Design review of the part built by this model. Coordinates are the model's own, in mm. Face numbers are marked on the shaded views. A direction names the side the tool comes from. Coordinates: 2 decimals unless noted, no trailing zeros. Write each loop counter-clockwise with the first axis right and the second up, starting at its lowest first coordinate (ties: lowest second). Pieces come first, ordered by that corner, then holes.
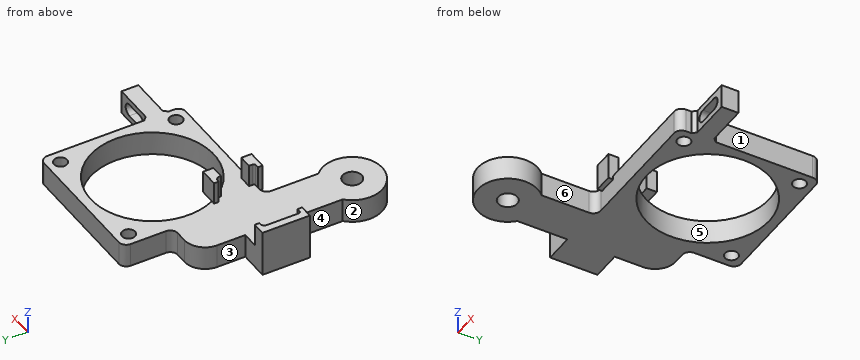
```python
from build123d import *
from OCP.BRepFilletAPI import BRepFilletAPI_MakeFillet

# Parameters (mm, degrees)
SKETCH1_R                 = 2.55
SKETCH1_R_2               = 1.75
SKETCH1_R_3               = 12.5
BOSS_EXTRUDE3_DEPTH       = 6.4
SKETCH1_5_R               = 2.55
BOSS_EXTRUDE2_DEPTH       = 1
CUT_EXTRUDE1_DEPTH        = 10
FILLET2_R                 = 2
CHAMFER2_SIZE             = 1
FILLET1_R                 = 2
SKETCH5_R                 = 16.5
CUT_EXTRUDE2_DEPTH        = 10
SKETCH6_W                 = 4.33
SKETCH6_H                 = 1.25
BOSS_EXTRUDE5_DEPTH       = 6.4
BOSS_EXTRUDE8_DEPTH       = 6
BOSS_EXTRUDE13_DEPTH      = 6
BOSS_EXTRUDE13_DEPTH_BACK = 1
FILLET3_R1                = 1
FILLET3_R2                = 0.5


with BuildPart() as part:
    # Sketch1 → Boss-Extrude3 (new body)
    with BuildSketch(Plane.XY):
        with BuildLine():
            ThreePointArc((-5.55, 5.830951895), (0, -8.05), (5.55, 5.830951895))
            Line((5.55, 5.830951895), (5.55, 20.5))
            Line((5.55, 20.5), (43, 20.5))
            Line((43, 20.5), (43, 25))
            Line((43, 25), (55, 25))
            Line((55, 25), (55, 29.5))
            Line((55, 29.5), (43, 29.5))
            Line((43, 29.5), (43, 58.5))
            Line((43, 58.5), (5, 58.5))
            Line((5, 58.5), (5, 45.05))
            Line((5, 45.05), (0, 45.05))
            ThreePointArc((0, 45.05), (-3.924442636, 43.424442636), (-5.55, 39.5))
            Line((-5.55, 39.5), (-5.55, 5.830951895))
        make_face()
        Circle(SKETCH1_R, mode=Mode.SUBTRACT)
        with Locations((39.5, 24)):
            Circle(SKETCH1_R_2, mode=Mode.SUBTRACT)
        with Locations((8.5, 55)):
            Circle(SKETCH1_R_2, mode=Mode.SUBTRACT)
        with Locations((24, 39.5)):
            Circle(SKETCH1_R_3, mode=Mode.SUBTRACT)
        with Locations((39.5, 55)):
            Circle(SKETCH1_R_2, mode=Mode.SUBTRACT)
    extrude(amount=BOSS_EXTRUDE3_DEPTH)

    # Sketch1<5> → Boss-Extrude2 (add)
    # profile 1 of 2: a face of its own
    with BuildSketch(Plane.XY):
        with BuildLine():
            Line((-5.55, 5.830951895), (-5.55, 0))
            ThreePointArc((-5.55, 0), (0, -5.55), (5.55, 0))
            Line((5.55, 0), (5.55, 5.830951895))
            ThreePointArc((5.55, 5.830951895), (0, 8.05), (-5.55, 5.830951895))
        make_face()
        Circle(SKETCH1_5_R, mode=Mode.SUBTRACT)
    # profile 2 of 2: a face of its own
    with BuildSketch(Plane.XY):
        with BuildLine():
            ThreePointArc((5.55, 0), (0, -5.55), (-5.55, 0))
            Line((-5.55, 0), (-5.55, 5.830951895))
            ThreePointArc((-5.55, 5.830951895), (-3.172144385, -7.398648525), (8.05, 0))
            ThreePointArc((8.05, 0), (7.398648525, 3.172144385), (5.55, 5.830951895))
            Line((5.55, 5.830951895), (5.55, 0))
        make_face()
    extrude(amount=BOSS_EXTRUDE2_DEPTH)

    # Sketch3 → Cut-Extrude1 (cut)
    with BuildSketch(Plane(origin=(0, 29.5, 0), x_dir=(1, 0, 0), z_dir=(0, 1, 0))):
        with BuildLine():
            Line((46.5, -1.55), (51.5, -1.55))
            ThreePointArc((51.5, -1.55), (53.15, -3.2), (51.5, -4.85))
            Line((51.5, -4.85), (46.5, -4.85))
            ThreePointArc((46.5, -4.85), (44.85, -3.2), (46.5, -1.55))
        make_face()
    extrude(amount=-CUT_EXTRUDE1_DEPTH, mode=Mode.SUBTRACT)

    # Fillet2
    fillet2_edges = [part.edges().sort_by_distance(p)[0] for p in [
        (5.55, 20.5, 3.2),
        (5, 45.05, 3.2),
    ]]
    fillet(fillet2_edges, radius=FILLET2_R)

    # Chamfer2
    chamfer2_edges = [part.edges().sort_by_distance(p)[0] for p in [
        (43, 29.5, 3.2),
        (43, 25, 3.2),
    ]]
    chamfer(chamfer2_edges, length=CHAMFER2_SIZE)

    # Fillet1
    fillet1_edges = [part.edges().sort_by_distance(p)[0] for p in [
        (43, 20.5, 3.2),
        (5, 58.5, 3.2),
        (43, 58.5, 3.2),
    ]]
    fillet(fillet1_edges, radius=FILLET1_R)

    # Sketch5 → Cut-Extrude2 (cut)
    with BuildSketch(Plane.XY.offset(6.4)):
        with Locations((24, 39.5)):
            Circle(SKETCH5_R)
    extrude(amount=-CUT_EXTRUDE2_DEPTH, mode=Mode.SUBTRACT)

    # Sketch6 → Boss-Extrude5 (add)
    with BuildSketch(Plane.XY.offset(6.4)):
        with Locations((-7.715, 31.325)):
            Rectangle(SKETCH6_W, SKETCH6_H)
        with BuildLine():
            Line((-5.55, 24.637668909), (-5.55, 30.45))
            Line((-5.55, 30.45), (-10.13, 30.45))
            ThreePointArc((-10.13, 30.45), (-10.837106781, 30.157106781), (-11.13, 29.45))
            Line((-11.13, 29.45), (-11.13, 21.25))
            ThreePointArc((-11.13, 21.25), (-10.983553391, 20.896446609), (-10.63, 20.75))
            Line((-10.63, 20.75), (-5.55, 20.75))
            Line((-5.55, 20.75), (-5.55, 21.862331091))
            ThreePointArc((-5.55, 21.862331091), (-7.525, 23.25), (-5.55, 24.637668909))
        make_face()
        with BuildLine():
            Line((-10.13, 30.45), (-5.55, 30.45))
            Line((-5.55, 30.45), (-5.55, 30.7))
            Line((-5.55, 30.7), (-9.88, 30.7))
            Line((-9.88, 30.7), (-11.38, 30.7))
            Line((-11.38, 30.7), (-11.38, 20.5))
            Line((-11.38, 20.5), (-9.88, 20.5))
            Line((-9.88, 20.5), (-5.55, 20.5))
            Line((-5.55, 20.5), (-5.55, 20.75))
            Line((-5.55, 20.75), (-10.63, 20.75))
            ThreePointArc((-10.63, 20.75), (-10.983553391, 20.896446609), (-11.13, 21.25))
            Line((-11.13, 21.25), (-11.13, 29.45))
            ThreePointArc((-11.13, 29.45), (-10.837106781, 30.157106781), (-10.13, 30.45))
        make_face()
        Polygon((-11.38, 30.7), (-9.88, 30.7), (-9.88, 31.95), (-13.38, 31.95), (-13.38, 19.25), (-9.88, 19.25), (-9.88, 20.5), (-11.38, 20.5), align=None)
        with Locations((-7.715, 19.875)):
            Rectangle(SKETCH6_W, SKETCH6_H)
        with BuildLine():
            Line((-5.55, 21.862331091), (-5.55, 24.637668909))
            ThreePointArc((-5.55, 24.637668909), (-7.525, 23.25), (-5.55, 21.862331091))
        make_face()
        with BuildLine():
            ThreePointArc((-4.575, 23.25), (-4.843118689, 24.09797553), (-5.55, 24.637668909))
            Line((-5.55, 24.637668909), (-5.55, 21.862331091))
            ThreePointArc((-5.55, 21.862331091), (-4.843118689, 22.40202447), (-4.575, 23.25))
        make_face()
    extrude(amount=-BOSS_EXTRUDE5_DEPTH)

    # Sketch6<4> → Boss-Extrude8 (add)
    with BuildSketch(Plane.XY.offset(6.4)):
        Polygon((-9.88, 30.7), (-9.88, 31.95), (-13.38, 31.95), (-13.38, 19.25), (-9.88, 19.25), (-9.88, 20.5), (-11.38, 20.5), (-11.38, 30.7), align=None)
        Polygon((8.17, 32.25), (8.17, 31), (9.67, 31), (9.67, 29.5), (13.17, 29.5), (13.17, 32.25), align=None)
    extrude(amount=BOSS_EXTRUDE8_DEPTH)

    # Sketch7 → Boss-Extrude13 (add, two sides: drawn at the far end of the back side and taken through both)
    with BuildSketch(Plane.XY.offset(6.4).offset(-BOSS_EXTRUDE13_DEPTH_BACK)):
        Polygon((9.67, 22), (9.67, 20.5), (8.17, 20.5), (8.17, 19.25), (13.17, 19.25), (13.17, 22), align=None)
    extrude(amount=BOSS_EXTRUDE13_DEPTH + BOSS_EXTRUDE13_DEPTH_BACK)

    # Fillet3: one fillet with a radius per group of edges: ONE call of the kernel's fillet builder (fillet() takes one radius for all edges)
    fillet3_edges_1 = [part.edges().sort_by_distance(p)[0] for p in [
        (-11.38, 30.7, 9.4),
        (9.67, 31, 9.4),
    ]]
    fillet3_edges_2 = [part.edges().sort_by_distance(p)[0] for p in [
        (9.67, 20.5, 9.4),
        (-11.38, 20.5, 9.4),
    ]]
    fillet3 = BRepFilletAPI_MakeFillet(part.part.solid().wrapped)
    for e in fillet3_edges_1:
        fillet3.Add(FILLET3_R1, e.wrapped)
    for e in fillet3_edges_2:
        fillet3.Add(FILLET3_R2, e.wrapped)
    add(Compound.cast(fillet3.Shape()), mode=Mode.REPLACE)


solid = part.part
```
(1) Mouldability with a two-part tool opening along X and no side actions: class the marked faces 4, 5 and 6 as +X half, -X half, draft (parallel to the pull), parting line (faces both ways), or undercut.
(2) Insertion check: pin 1 Ø0.5 at (x, z) = (-10.5, 10.5) entering from +Y; pin 2 Ø3 at (x, y) = (39.5, 24) entering from -Z; pin 3 Ø8 at (x, y) = (-4.5, 26.5) entering from +Z; pin 4 Ø5 at (y, z) = (40, 3.5) entering from -X. Each pin has a flat end and moves straight along its axis. Give the tip position at first contact, or say it passes through.
(3) Consider section B-B (z = 9). Give the boundary of the cut face in (x, y).
(4) For the marked faces 1, 2 and 3, list the 3-axis set-ups (+Z, -Z, +X, -X, +Y, -Y) from which the entire face can be reached by the end or side of a thin tool; tool diameter is ignored.
(5) Wall thickness on line 1 (X direction, y = 21.5, z = 9.75); line 2 (Y direction, x = 24, z = 2); line 3 (X direction, y = 39.5, z = 2.75): over which ranges is each line inside the solid? List them lowest first.
(6) Consider section C-C (x = 34). Give the boundary of the cut face in (y, z).
(7) Consider section A-A (y = 0). Give the boundary of the cut face in (x, z).
(8) Consider section D-D (y = 55). Give the boundary of the cut face in (x, z).
Results:
1. face 4: -X half
1. face 5: undercut
1. face 6: +X half
2. pin 1: stops at y = 31.95
2. pin 2: passes through
2. pin 3: stops at z = 6.4
2. pin 4: stops at x = -5.55
3. outline: (-13.38, 19.25) - (-9.88, 19.25) - (-9.88, 20.5) - (-10.88, 20.5) arc R0.5 cw to (-11.38, 21) - (-11.38, 29.7) arc R1 cw to (-10.38, 30.7) - (-9.88, 30.7) - (-9.88, 31.95) - (-13.38, 31.95) - close; (8.17, 19.25) - (13.17, 19.25) - (13.17, 22) - (9.67, 22) - (9.67, 21) arc R0.5 cw to (9.17, 20.5) - (8.17, 20.5) - close; (8.17, 31) - (8.67, 31) arc R1 cw to (9.67, 30) - (9.67, 29.5) - (13.17, 29.5) - (13.17, 32.25) - (8.17, 32.25) - close
4. face 1: +Z, -Z, +X, +Y
4. face 2: +Z, -Z
4. face 3: +Z, -Z, -X, +Y
5. line 1: x = -13.38 to -11.38, 9.67 to 13.17
5. line 2: y = 20.5 to 23, 56 to 58.5
5. line 3: x = -5.55 to 7.5, 40.5 to 43
6. outline: (20.5, 0) - (26.38, 0) - (26.38, 6.4) - (20.5, 6.4) - close; (52.62, 0) - (58.5, 0) - (58.5, 6.4) - (52.62, 6.4) - close
7. outline: (-8.05, 0) - (-2.55, 0) - (-2.55, 6.4) - (-8.05, 6.4) - close; (2.55, 0) - (8.05, 0) - (8.05, 6.4) - (2.55, 6.4) - close
8. outline: (5, 0) - (6.75, 0) - (6.75, 6.4) - (5, 6.4) - close; (10.25, 0) - (18.34, 0) - (18.34, 6.4) - (10.25, 6.4) - close; (29.66, 0) - (37.75, 0) - (37.75, 6.4) - (29.66, 6.4) - close; (41.25, 0) - (43, 0) - (43, 6.4) - (41.25, 6.4) - close
